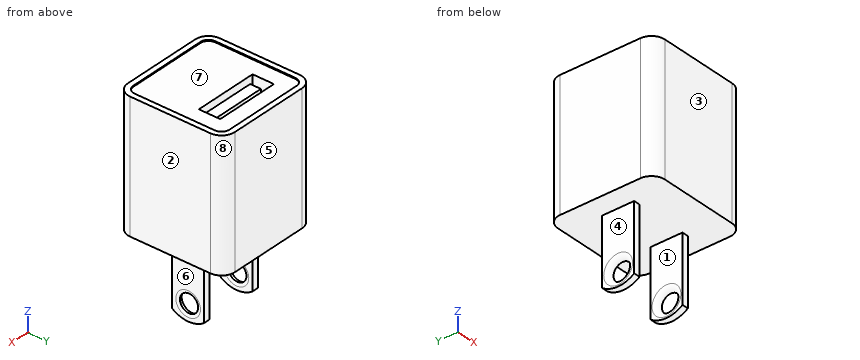
Autodesk Inventor part; units mm, degrees
ref_plane "YZ Plane" through (0, 0, 0) normal (1, 0, 0) x (0, 1, 0)
ref_plane "XZ Plane" through (0, 0, 0) normal (0, 1, 0) x (-1, 0, 0)
ref_plane "XY Plane" through (0, 0, 0) normal (0, 0, 1) x (1, 0, 0)
sketch "Sketch1" plane through (0, 0, 0) normal (0, 0, 1) x (1, 0, 0)
  line L0 (-12.7, -12.7) -> (12.7, -12.7)
  line L1 (12.7, -12.7) -> (12.7, 12.7)
  line L2 (12.7, 12.7) -> (-12.7, 12.7)
  line L3 (-12.7, 12.7) -> (-12.7, -12.7)
  line L4 (-12.7, -12.7) -> (12.7, 12.7) construction
  line L5 (12.7, -12.7) -> (-12.7, 12.7) construction
  point P0 (0, 0)
  dimension "d0" = 25.4
extrude "Extrusion1" add sketch "Sketch1" along normal blind 30.48
fillet "Fillet1" radius 3.175 4 edges at (-12.7, 12.7, 15.24) (-12.7, -12.7, 15.24) (12.7, -12.7, 15.24) (12.7, 12.7, 15.24)
sketch "Sketch2" plane through (0, 0, 30.48) normal (0, 0, 1) x (1, 0, 0)
  arc A0 (12.7, 9.525) -> (9.525, 12.7) centre (9.525, 9.525) ccw
  line L0 (9.525, 12.7) -> (-9.525, 12.7)
  arc A1 (-9.525, 12.7) -> (-12.7, 9.525) centre (-9.525, 9.525) ccw
  line L1 (-12.7, 9.525) -> (-12.7, -9.525)
  arc A2 (-12.7, -9.525) -> (-9.525, -12.7) centre (-9.525, -9.525) ccw
  line L2 (-9.525, -12.7) -> (9.525, -12.7)
  arc A3 (9.525, -12.7) -> (12.7, -9.525) centre (9.525, -9.525) ccw
  line L3 (12.7, -9.525) -> (12.7, 9.525)
  line L4 (-9.525, 11.43) -> (9.525, 11.43)
  arc A4 (11.43, 9.525) -> (9.525, 11.43) centre (9.525, 9.525) ccw
  line L5 (11.43, 9.525) -> (11.43, -9.525)
  arc A5 (9.525, -11.43) -> (11.43, -9.525) centre (9.525, -9.525) ccw
  line L6 (9.525, -11.43) -> (-9.525, -11.43)
  arc A6 (-11.43, -9.525) -> (-9.525, -11.43) centre (-9.525, -9.525) ccw
  line L7 (-11.43, -9.525) -> (-11.43, 9.525)
  arc A7 (-9.525, 11.43) -> (-11.43, 9.525) centre (-9.525, 9.525) ccw
  point P0 (0, 0)
  dimension "d4" = 1.27
extrude "Extrusion2" cut sketch "Sketch2" against normal blind 0.254 contours L4 A4 L5 A5 L6 A6 L7 A7
sketch "Sketch3" plane through (0, 0, 30.226) normal (0, 0, 1) x (1, 0, 0)
  line L0 (-7.62, 7.62) -> (7.62, 7.62)
  line L1 (7.62, 7.62) -> (7.62, 2.54)
  line L2 (7.62, 2.54) -> (-7.62, 2.54)
  line L3 (-7.62, 2.54) -> (-7.62, 7.62)
  line L4 (-7.62, 7.62) -> (7.62, 2.54) construction
  line L5 (7.62, 7.62) -> (-7.62, 2.54) construction
  line L6 (11.43, 9.525) -> (11.43, -9.525)
  line L7 (-11.43, -9.525) -> (-11.43, 9.525)
  line L8 (-9.525, 11.43) -> (9.525, 11.43)
  point P0 (0, 0)
  point P1 (0, 5.08)
  dimension "d7" = 3.81
  dimension "d8" = 3.81
  dimension "d9" = 3.81
  dimension "d10" = 5.08
extrude "Extrusion3" cut sketch "Sketch3" against normal blind 10.16
sketch "Sketch4" plane through (0, 0, 20.066) normal (0, 0, 1) x (1, 0, 0)
  line L0 (-6.35, 5.588) -> (6.35, 5.588)
  line L1 (6.35, 5.588) -> (6.35, 3.048)
  line L2 (6.35, 3.048) -> (-6.35, 3.048)
  line L3 (-6.35, 3.048) -> (-6.35, 5.588)
  line L4 (-6.35, 5.588) -> (6.35, 3.048) construction
  line L5 (6.35, 5.588) -> (-6.35, 3.048) construction
  line L6 (-7.62, 2.54) -> (-7.62, 7.62)
  line L7 (7.62, 7.62) -> (7.62, 2.54)
  line L8 (7.62, 2.54) -> (-7.62, 2.54)
  point P0 (0, 0)
  point P1 (0, 4.318)
  point P2 (7.62, 5.08)
  dimension "d13" = 1.27
  dimension "d14" = 1.27
  dimension "d15" = 0.508
  dimension "d16" = 2.54
extrude "Extrusion4" add sketch "Sketch4" along normal blind 8.89
sketch "Sketch5" plane through (0, 0, 0) normal (0, 0, -1) x (-1, 0, 0)
  line L0 (0, 0) -> (6.858, 0) construction
  line L1 (0, 0) -> (-6.858, 0) construction
  line L2 (6.096, -3.81) -> (7.62, -3.81)
  line L3 (7.62, -3.81) -> (7.62, 3.81)
  line L4 (7.62, 3.81) -> (6.096, 3.81)
  line L5 (6.096, 3.81) -> (6.096, -3.81)
  line L6 (6.096, -3.81) -> (7.62, 3.81) construction
  line L7 (7.62, -3.81) -> (6.096, 3.81) construction
  line L8 (-7.62, -3.81) -> (-6.096, -3.81)
  line L9 (-6.096, -3.81) -> (-6.096, 3.81)
  line L10 (-6.096, 3.81) -> (-7.62, 3.81)
  line L11 (-7.62, 3.81) -> (-7.62, -3.81)
  line L12 (-7.62, -3.81) -> (-6.096, 3.81) construction
  line L13 (-6.096, -3.81) -> (-7.62, 3.81) construction
  dimension "d19" = 6.858
  dimension "d20" = 7.62
  dimension "d21" = 1.524
extrude "Extrusion5" add sketch "Sketch5" along normal blind 17.78
sketch "Sketch6" plane through (-7.62, -3.81, 0) normal (-1, 0, 0) x (0, 0, 1)
  line L0 (0, 7.62) -> (-17.78, 7.62)
  line L1 (0, 0) -> (-17.78, 0)
  arc A0 (-15.748, 7.62) -> (-15.748, 0) centre (-10.668, 3.81) ccw
  line L2 (-15.748, 7.62) -> (-17.78, 7.62)
  line L3 (-17.78, 0) -> (-17.78, 7.62)
  line L4 (-17.78, 0) -> (-15.748, 0)
  point P0 (0, 3.81)
  dimension "d24" = 2.032
  dimension "d25" = 2.032
  dimension "d26" = 6.35
extrude "Extrusion6" cut sketch "Sketch6" against normal blind 17.78
sketch "Sketch7" plane through (-7.62, -3.81, 0) normal (-1, 0, 0) x (0, 0, 1)
  arc A0 (-15.748, 7.62) -> (-15.748, 0) centre (-10.668, 3.81) ccw construction
  line L0 (-17.018, 3.81) -> (-13.208, 3.81) construction
  circle A1 centre (-13.208, 3.81) radius 2.159
  point P0 (0, 3.81)
  dimension "d29" = 3.81
  dimension "d30" = 4.318
extrude "Extrusion7" cut sketch "Sketch7" against normal blind 17.78
fillet "Fillet2" radius 1.27 4 edges at (-7.62, 0, -15.367) (6.096, 0, -15.367) (-6.096, 0, -15.367) (7.62, 0, -15.367)
properties part number "iPhone Charger"
Design review of the part built by this model. Coordinates are the model's own, in mm. Face numbers are marked on the shaded views. A direction names the side the tool comes from. Coordinates: 2 decimals unless noted, no trailing zeros. Order: outer loops, then holes, each group sorted by start corner. A loop starts at its lowest first (then second) coordinate and runs counter-clockwise, first axis right, second up.
Item 1: Take a section at C-C, the plane y = -10.5. Write out the cut boundary in (x, z), then the cut area to 3 significant figures.
Item 2: Take a section at A-A, the plane z = 22. Write out the cut boundary in (x, y) (3 decimals).
Item 3: For line 1 (Y direction, x = -3.75, z = 27); line 2 (Z direction, x = 11, y = 10.25); line 3 (X direction, y = -3.75, z = -10), list the stretches that pass through material, from the lowest coordinate up.
Item 4: Take a section at D-D, the plane x = -2.5. Write out the cut boundary in (y, z).
Item 5: Take a section at B-B, the plane x = -8.75. Write out the cut boundary in (y, z), then the cut area to 3 significant figures.
Item 6: The part is to be moulded in two halves that separate along X. For the marked faces 1, 2 and 3, say which applies: pulls with the +X half, pulls with the -X half, needs draft (parallel to the pull), parting line crosses it, or undercut.
Item 7: For the marked faces 4, 5, 6, 7 and 8, list the 3-axis set-ups (+Z, -Z, +X, -X, +Y, -Y) from which the entire face can be reached by the end or side of a thin tool; tool diameter is ignored.
Item 8: For pin 1 Ø8.5 at (y, z) = (-1, -6) entering from +X; pin 2 Ø11.5 at (x, y) = (-3, 0.5) entering from +Z; pin 3 Ø6 at (y, z) = (9, -7.5) entering from -X; pin 4 Ø1.7 at (x, z) = (-6.5, -6) entering from -Y, all flat-tipped, find the tip position at first contact; note any pin that passes through.
The answers:
1. outline: (-12.55, 0) - (12.55, 0) - (12.55, 30.48) - (11.16, 30.48) - (11.16, 30.23) - (-11.16, 30.23) - (-11.16, 30.48) - (-12.55, 30.48) - close
1. area: 759 mm2
2. outline: (-12.7, -9.525) arc R3.175 ccw to (-9.525, -12.7) - (9.525, -12.7) arc R3.175 ccw to (12.7, -9.525) - (12.7, 9.525) arc R3.175 ccw to (9.525, 12.7) - (-9.525, 12.7) arc R3.175 ccw to (-12.7, 9.525) - close; (-6.35, 3.048) - (6.35, 3.048) - (6.35, 5.588) - (-6.35, 5.588) - close; hole (-7.62, 2.54) - (7.62, 2.54) - (7.62, 7.62) - (-7.62, 7.62) - close
3. line 1: y = -12.7 to 2.54, 3.05 to 5.59, 7.62 to 12.7
3. line 2: z = 0 to 30.23
3. line 3: x = -7.62 to -6.1, 6.1 to 7.62
4. outline: (-12.7, 0) - (12.7, 0) - (12.7, 30.48) - (11.43, 30.48) - (11.43, 30.23) - (7.62, 30.23) - (7.62, 20.07) - (5.59, 20.07) - (5.59, 28.96) - (3.05, 28.96) - (3.05, 20.07) - (2.54, 20.07) - (2.54, 30.23) - (-11.43, 30.23) - (-11.43, 30.48) - (-12.7, 30.48) - close
5. outline: (-12.7, 0) - (12.7, 0) - (12.7, 30.48) - (11.43, 30.48) - (11.43, 30.23) - (-11.43, 30.23) - (-11.43, 30.48) - (-12.7, 30.48) - close
5. area: 768 mm2
6. face 1: undercut
6. face 2: pulls with the +X half
6. face 3: needs draft
7. face 4: -Z, -X, +Y, -Y
7. face 5: +Z, -Z, +X, -X, +Y
7. face 6: -Z, +X, +Y, -Y
7. face 7: +Z
7. face 8: +Z, -Z, +X, +Y
8. pin 1: stops at x = 7.62
8. pin 2: stops at z = 30.23
8. pin 3: passes through
8. pin 4: stops at y = -3.81
